```python
from build123d import *

# Parameters (mm, degrees)
SKETCH1_W           = 2
SKETCH1_H           = 4
SKETCH2_R           = 2.5
BOSS_EXTRUDE1_DEPTH = 6
SKETCH3_R           = 1.5
BOSS_EXTRUDE2_DEPTH = 10
CUT_EXTRUDE1_DEPTH  = 2
CHAMFER1_SIZE       = 0.3065


with BuildPart() as part:
    # Sketch1 → Revolve1 (revolve)
    with BuildSketch(Plane.XY, mode=Mode.PRIVATE) as revolve1_sk:
        with Locations((-7, 2)):
            Rectangle(SKETCH1_W, SKETCH1_H)
    revolve(revolve1_sk.sketch.rotate(Axis((-8, 0, 0), (1, 0, 0)), 270), axis=Axis((-8, 0, 0), (1, 0, 0)))

    # Sketch2 → Boss-Extrude1 (add)
    with BuildSketch(Plane(origin=(-6, 0, 0), x_dir=(0, 0, -1), z_dir=(1, 0, 0))):
        Circle(SKETCH2_R)
    extrude(amount=BOSS_EXTRUDE1_DEPTH)

    # Sketch3 → Boss-Extrude2 (add)
    with BuildSketch(Plane(origin=(0, 0, 0), x_dir=(0, 0, -1), z_dir=(1, 0, 0))):
        Circle(SKETCH3_R)
    extrude(amount=BOSS_EXTRUDE2_DEPTH)

    # Sketch4 → Cut-Extrude1 (cut)
    with BuildSketch(Plane.ZY.offset(8)):
        Polygon((0, -1.154700538), (1, -0.577350269), (1, 0.577350269), (0, 1.154700538), (-1, 0.577350269), (-1, -0.577350269), align=None)
    extrude(amount=-CUT_EXTRUDE1_DEPTH, mode=Mode.SUBTRACT)

    # Sketch5 → Cut-Revolve1 (revolve, cut)
    with BuildSketch(Plane.XY, mode=Mode.PRIVATE) as cut_revolve1_sk:
        Polygon((-6, 1), (-6, 0), (-5.422649731, 0), align=None)
    revolve(cut_revolve1_sk.sketch.rotate(Axis((-6.000025, 0, 0), (1, 0, 0)), 90), axis=Axis((-6.000025, 0, 0), (1, 0, 0)), mode=Mode.SUBTRACT)

    # Chamfer1
    chamfer1_edges = [part.edges().sort_by_distance(p)[0] for p in [
        (10, 0, 1.5),
    ]]
    chamfer(chamfer1_edges, length=CHAMFER1_SIZE)


solid = part.part
```
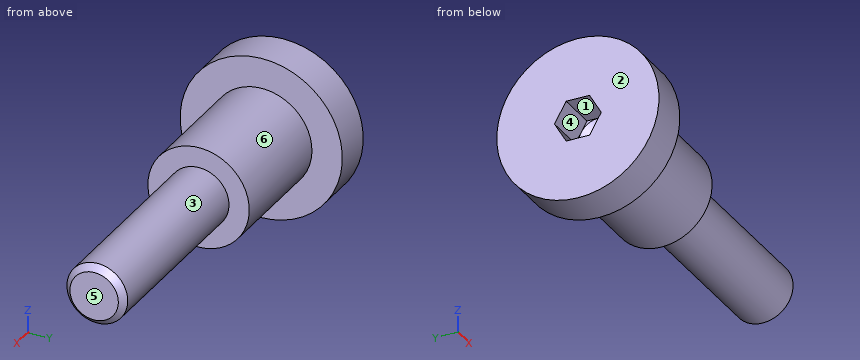
Check sheet for the modelled part. Datum: model origin and axes. Units: mm. Face numbers are marked on the shaded views. A direction names the side the tool comes from. Coordinates: 2 decimals unless noted, no trailing zeros. Write each loop counter-clockwise with the first axis right and the second up, starting at its lowest first coordinate (ties: lowest second). Pieces come first, ordered by that corner, then holes. Notation, with made-up numbers: (32.25, 28.25) - (87.25, 28.25) arc R20 cw to (87.25, 58.25) - close; hole circle Ø6 at (22.25, 4). An arc over 180 degrees is marked (long way). One line per question, with ' | ' between items.
Item 1: Sectioned sample at C-C on z = 3.25. Record the boundary of the cut face in (x, y), plus the area to 3 significant figures.
Determined:
outline: (-8, -2.33) - (-6, -2.33) - (-6, 2.33) - (-8, 2.33) - close | area: 9.33 mm2
Item 2: Sectioned sample at B-B on x = 7.25. Record the boundary of the cut face in (y, z), plus the area to 3 significant figures.
Determined:
outline: circle Ø3 at (0, 0) | area: 7.07 mm2
Item 3: Gauge pin test, flat ends, axial feed: P1, Ø3, axis at y = 1.5, z = -2.5, coming from the +X side; P2, Ø4, axis at y = 0, z = -2.5, coming from the +X side; P3, Ø4, axis at x = 4, y = 0.5, coming from the -Z side. Record the tip position at first contact, or that the pin passes through.
Determined:
P1: stops at x = 9.78 | P2: stops at x = 10 | P3: stops at z = -1.5
Item 4: Sectioned sample at D-D on y = 3. Record the boundary of the cut face in (x, z), plus the area to 3 significant figures.
Determined:
outline: (-8, -2.65) - (-6, -2.65) - (-6, 2.65) - (-8, 2.65) - close | area: 10.6 mm2
Item 5: Mould release check, pull along Z, two halves, no side actions. Record for the marked faces 1, 2 and 3: pulls with the +Z half, pulls with the -Z half, needs draft (parallel to the pull), parting line crosses it, or undercut.
Determined:
face 1: undercut | face 2: needs draft | face 3: parting line crosses it
Item 6: Access from +Z, -Z, +X, -X, +Y, -Y to the whole of each face (thin tool, end or side, straight path). Record for the marked faces 4, 5 and 6.
Determined:
face 4: -X | face 5: +Z, -Z, +X, +Y, -Y | face 6: +X
Item 7: Thickness scan on line 1 (X direction, y = 0, z = -2.25); line 2 (Y direction, x = -7, z = 0.25); line 3 (X direction, y = 1.5, z = -3.5). Record the ranges inside material, lowest first. Write a range as [from, to].
Determined:
line 1: x = [-8, 0] | line 2: y = [-3.99, -1.01], [1.01, 3.99] | line 3: x = [-8, -6]
Item 8: Sectioned sample at A-A on y = -2.25. Record the boundary of the cut face in (x, z), plus the area to 3 significant figures.
Determined:
outline: (-8, -3.31) - (-6, -3.31) - (-6, -1.09) - (0, -1.09) - (0, 1.09) - (-6, 1.09) - (-6, 3.31) - (-8, 3.31) - close | area: 26.3 mm2
